from build123d import *

# Parameters (mm, degrees)
F1_DEPTH = 71
F3_DEPTH = 71
F5_DEPTH = 71


with BuildPart() as f1:
    # F0 (on Front) → F1 (new body)
    with BuildSketch(Plane.XZ):
        Polygon((8.899987, -0.01517), (4.463131, 7.70003), (-4.436856, 7.7152), (-8.899987, 0.01517), (-4.463131, -7.70003), (4.436856, -7.7152), align=None)
    extrude(amount=F1_DEPTH)

    # F2 (on face) → F3 (cut)
    with BuildSketch(Plane.XZ.offset(71)):
        Polygon((8.899987, -0.01517), (-8.899987, 0.01517), (-4.463131, -7.70003), (4.436856, -7.7152), align=None)
    extrude(amount=-F3_DEPTH, mode=Mode.SUBTRACT)

    # F4 (on face) → F5 (cut)
    with BuildSketch(Plane(origin=(0, 0, 0), x_dir=(-1, 0, 0), z_dir=(0, 1, 0))):
        Polygon((-5.549992, 5.8101), (-8.899987, -0.01517), (-5.549992, -0.00946), align=None)
        Polygon((5.549992, 0.00946), (8.899987, 0.01517), (5.549992, 5.794759), align=None)
    extrude(amount=-F5_DEPTH, mode=Mode.SUBTRACT)


solid = f1.part
Design review of the part built by this model. Coordinates are the model's own, in mm. Give positions to 0.01 mm unless a question says otherwise; leave off trailing zeros. Loops run counter-clockwise (first coordinate to the right, second up) from the corner with the lowest first, then second, coordinate; pieces in that order, holes last. Notation, with made-up numbers: (-17.75, 67.25) - (21.25, 67.25) arc R22 ccw to (21.25, 98.25) - close; hole circle Ø8 at (-24, 17.25). An arc over 180 degrees is marked (long way). Use CSV: the item, a comma, the result in double quotes. Start each with the question number.
1. Add section A-A (y = -53). State the section outline as (x, z) points.
2. Add section B-B (z = 7). State the section outline as (x, y) points, plus the area to 3 significant figures.
3. Insertion check: P1, Ø2, axis at x = -4, y = -30, coming from the -Z side; P2, Ø2, axis at x = 0.5, y = -30.5, coming from the +Z side; P3, Ø1, axis at y = -25, z = 6.5, coming from the +X side. Each pin has a flat end and moves straight along its axis. Give the tip position at first contact, or say it passes through.
4. Wall thickness on L1, parallel to Z at x = -0.75, y = -52.5; L2, parallel to X at y = -33, z = 7.25; L3, parallel to Z at x = -4.5, y = -13: over which ranges is each line inside the solid? List them lowest first.
Results found:
1,outline,"(-5.55, 0.01) - (5.55, -0.01) - (5.55, 5.81) - (4.46, 7.7) - (-4.44, 7.72) - (-5.55, 5.79) - close"
2,outline,"(-4.85, -71) - (4.87, -71) - (4.87, 0) - (-4.85, 0) - close"
2,area,"690 mm²"
3,P1,"stops at z = 0.01"
3,P2,"stops at z = 7.71"
3,P3,"stops at x = 5.44"
4,L1,"z = 0 to 7.71"
4,L2,"x = -4.71 to 4.72"
4,L3,"z = 0.01 to 7.61"
